Build history of the part. All positions in model axes, mm. Face numbers are marked on the shaded views. A direction names the side the tool comes from. Coordinates: 2 decimals unless noted, no trailing zeros. Loops run counter-clockwise (first coordinate to the right, second up) from the corner with the lowest first, then second, coordinate; pieces in that order, holes last. Notation, with made-up numbers: (82.25, -20) -> (122.25, -20) arc R10 cw to (122.25, -14) -> close; hole circle Ø1 at (-24.75, -35). An arc over 180 degrees is marked (long way). One line per item, written item: value. Start each with the question number.
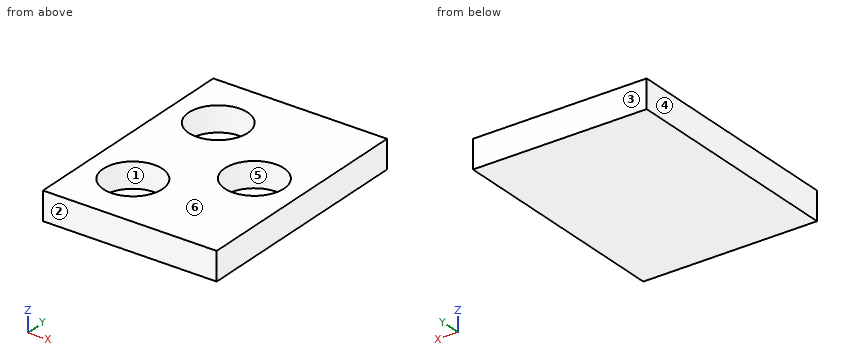
```python
from build123d import *

# Parameters (mm, degrees)
F0_W     = 276.5
F0_H     = 373
F2_DEPTH = 45
F1_R     = 47
F3_DEPTH = 40


with BuildPart() as f2:
    # F0 (on Top) → F2 (new body)
    with BuildSketch(Plane.XY):
        Rectangle(F0_W, F0_H)
    extrude(amount=-F2_DEPTH)

    # F1 (on face) → F3 (cut)
    with BuildSketch(Plane.XY):
        with Locations((-63.016894, 93.755925)):
            Circle(F1_R)
        with Locations((62.786135, -0.109312)):
            Circle(F1_R)
        with Locations((-63.016894, -93.244075)):
            Circle(F1_R)
    extrude(amount=-F3_DEPTH, mode=Mode.SUBTRACT)


solid = f2.part
```
Item 1: Two-plate mould, pull along Y, no slides. Class the marked faces 1, 2, 3 and 4: +Y half, -Y half, draft (parallel to the pull), parting line (faces both ways), or undercut.
Item 2: Band-saw the part on D-D, the plane y = 103. List the corners of the cut face in (x, z).
Item 3: Band-saw the part on B-B, the plane x = -73. List the corners of the cut face in (y, z).
Item 4: Band-saw the part on C-C, the plane z = -5.5. List the corners of the cut face in (x, y).
Item 5: Probe probe 1 along Y at (x, z) = (-58.5, -23); probe 2 along Y at (x, z) = (-80, -27); probe 3 along Z at (x, y) = (-25.5, 86). List the from-to ranges inside material, lowest first.
Item 6: Drop a flat-ended pin along its axis: pin 1 Ø6 at (x, y) = (104.5, 10) entering from +Z. Give the stop position or say it passes through.
Item 7: Tool access for the marked faces 5 and 6: list every direction of +Z, -Z, +X, -X, +Y, -Y with a clear straight run to the whole face (end or side of a thin tool).
Item 8: Band-saw the part on A-A, the plane y = -35. List the corners of the cut face in (x, z).
Worked out:
1. face 1: undercut
1. face 2: -Y half
1. face 3: +Y half
1. face 4: draft
2. outline: (-138.25, -45) -> (138.25, -45) -> (138.25, 0) -> (-16.93, 0) -> (-16.93, -40) -> (-109.1, -40) -> (-109.1, 0) -> (-138.25, 0) -> close
3. outline: (-186.5, -45) -> (186.5, -45) -> (186.5, 0) -> (139.68, 0) -> (139.68, -40) -> (47.83, -40) -> (47.83, 0) -> (-47.32, 0) -> (-47.32, -40) -> (-139.17, -40) -> (-139.17, 0) -> (-186.5, 0) -> close
4. outline: (-138.25, -186.5) -> (138.25, -186.5) -> (138.25, 186.5) -> (-138.25, 186.5) -> close; hole circle Ø94 at (-63.02, -93.24); hole circle Ø94 at (-63.02, 93.76); hole circle Ø94 at (62.79, -0.11)
5. probe 1: y = -186.5 to -140.03, -46.46 to 46.97, 140.54 to 186.5
5. probe 2: y = -186.5 to -137.07, -49.42 to 49.93, 137.58 to 186.5
5. probe 3: z = -45 to -40
6. pin 1: stops at z = -40
7. face 5: +Z
7. face 6: +Z, +X, -X, +Y, -Y
8. outline: (-138.25, -45) -> (138.25, -45) -> (138.25, 0) -> (94.28, 0) -> (94.28, -40) -> (31.3, -40) -> (31.3, 0) -> (-138.25, 0) -> close
